from build123d import *

# Parameters (mm, degrees)
SKETCH1_W           = 75
SKETCH1_H           = 75
BOSS_EXTRUDE1_DEPTH = 12.7
FILLET1_R           = 7
CUT_EXTRUDE1_REACH  = 56.532
SKETCH2_R           = 25.4254
CUT_EXTRUDE2_REACH  = 56.532
SKETCH3_R           = 4.165
CIRPATTERN1_COUNT   = 4


with BuildPart() as part:
    # Sketch1 → Boss-Extrude1 (new body)
    with BuildSketch(Plane.XY):
        Rectangle(SKETCH1_W, SKETCH1_H)
    extrude(amount=BOSS_EXTRUDE1_DEPTH)

    # Fillet1
    fillet1_edges = [part.edges().sort_by_distance(p)[0] for p in [
        (37.5, -37.5, 6.35),
        (-37.5, -37.5, 6.35),
        (-37.5, 37.5, 6.35),
        (37.5, 37.5, 6.35),
    ]]
    fillet(fillet1_edges, radius=FILLET1_R)

    # Sketch2 → Cut-Extrude1 (cut, up to next)
    with BuildSketch(Plane.XY.offset(12.7), mode=Mode.PRIVATE) as cut_extrude1_sk1:
        Circle(SKETCH2_R)
    cut_extrude1_tool1 = extrude(cut_extrude1_sk1.sketch, amount=-CUT_EXTRUDE1_REACH, mode=Mode.PRIVATE) & part.part
    add(cut_extrude1_tool1.solids().sort_by_distance((0, 0, 12.7))[0], mode=Mode.SUBTRACT)

    # Sketch3 → Cut-Extrude2 (cut, up to next)
    with BuildSketch(Plane.XY.offset(12.7), mode=Mode.PRIVATE) as cut_extrude2_sk1:
        with Locations((-30, 30)):
            Circle(SKETCH3_R)
    cut_extrude2_tool1 = extrude(cut_extrude2_sk1.sketch, amount=-CUT_EXTRUDE2_REACH, mode=Mode.PRIVATE) & part.part
    cut_extrude2 = cut_extrude2_tool1.solids().sort_by_distance((-30, 30, 12.7))[0]
    add(cut_extrude2, mode=Mode.SUBTRACT)

    # CirPattern1: Cut-Extrude2 ×4 about axis
    cirpattern1_axis = Axis((0, 0, 0), (0, 0, 1))
    for i in range(1, CIRPATTERN1_COUNT):
        add(cut_extrude2.rotate(cirpattern1_axis, i * 360 / CIRPATTERN1_COUNT), mode=Mode.SUBTRACT)


solid = part.part
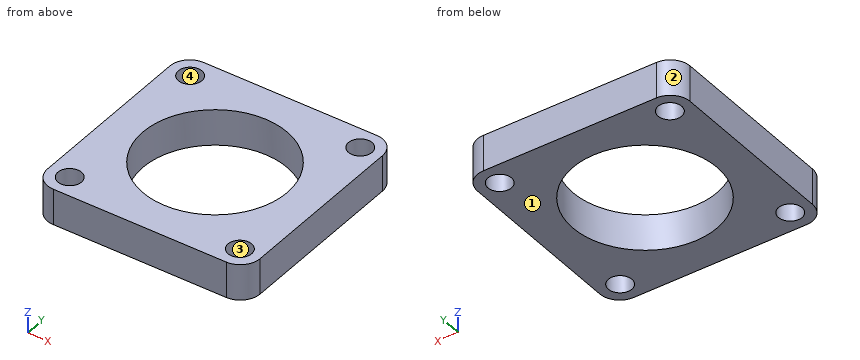
For this review, take the finished solid that the model builds, in its own axes (mm). Face numbers are marked on the shaded views. Give positions to 0.01 mm unless a question says otherwise; leave off trailing zeros. Order: outer loops, then holes, each group sorted by start corner. A loop starts at its lowest first (then second) coordinate and runs counter-clockwise, first axis right, second up. Notation, with made-up numbers: M -2,-6.5 L 43,-6.5 A17 cw 43,25.5 Z; hole C 57.5,78.5 d2. An arc over 180 degrees is marked long. Answer in a Markdown table with one row per item. Add a question column.
(1) Wall thickness on probe 1 along Y at (x, z) = (-30, 9.5) (3 decimals); probe 2 along X at (y, z) = (0.5, 7.25): over which ranges is each line inside the solid? List them lowest first. Write a range as [from, to].
(2) Mouldability with a two-part tool opening along Y and no side actions: class the marked faces 1, 2, 3 and 4 as +Y half, -Y half, draft (parallel to the pull), parting line (faces both ways), or undercut.
(3) For pin 1 (11 mm diameter, centred on x = 30, y = 30, fed in from +Z), flat-tipped, find the tip position at first contact; note if it passes through.
(4) Consider section B-B on z = 11.25. State the section outline as (x, y) points (3 decimals), and give its area (3 significant figures).
(5) Consider section C-C on y = 21. State the section outline as (x, z) points, and give its area (3 significant figures).
(6) Consider section A-A on x = 0. State the section outline as (y, z) points, and give its area (3 significant figures).
Evaluation:
| question | item | result |
|---|---|---|
| 1 | probe 1 | y = [-37.5, -34.165], [-25.835, 25.835], [34.165, 37.5] |
| 1 | probe 2 | x = [-37.5, -25.42], [25.42, 37.5] |
| 2 | face 1 | draft |
| 2 | face 2 | +Y half |
| 2 | face 3 | undercut |
| 2 | face 4 | undercut |
| 3 | pin 1 | stops at z = 12.7 |
| 4 | outline | M -37.5,-30.5 A7 ccw -30.5,-37.5 L 30.5,-37.5 A7 ccw 37.5,-30.5 L 37.5,30.5 A7 ccw 30.5,37.5 L -30.5,37.5 A7 ccw -37.5,30.5 Z; hole C -30,-30 d8.33; hole C -30,30 d8.33; hole C 0,0 d50.851; hole C 30,-30 d8.33; hole C 30,30 d8.33 |
| 4 | area | 3,330 mm^2 |
| 5 | outline | M -37.5,0 L -14.33,0 L -14.33,12.7 L -37.5,12.7 Z; M 14.33,0 L 37.5,0 L 37.5,12.7 L 14.33,12.7 Z |
| 5 | area | 588 mm^2 |
| 6 | outline | M -37.5,0 L -25.43,0 L -25.43,12.7 L -37.5,12.7 Z; M 25.43,0 L 37.5,0 L 37.5,12.7 L 25.43,12.7 Z |
| 6 | area | 307 mm^2 |
